Check sheet for the modelled part. Datum: model origin and axes. Units: mm. Face numbers are marked on the shaded views. A direction names the side the tool comes from. Give positions to 0.01 mm unless a question says otherwise; leave off trailing zeros. Loops run counter-clockwise (first coordinate to the right, second up) from the corner with the lowest first, then second, coordinate; pieces in that order, holes last. Notation, with made-up numbers: M -39.5,31.25 L -21.5,31.25 A20 cw -21.5,47.25 Z; hole C 31.25,-25.5 d1. An arc over 180 degrees is marked long. One line per question, with ' | ' between items. Start each with the question number.
from build123d import *

# Parameters (mm, degrees)
EXTRUDE_THIN1_DEPTH = 2.921
FILLET1_R           = 1.27
SKETCH2_W           = 6.858
SKETCH2_H           = 2.6035
CUT_EXTRUDE1_DEPTH  = 23.45746426


with BuildPart() as part:
    # Sketch1 → Extrude-Thin1 (new, symmetric)
    with BuildSketch(Plane(origin=(0, 0, 0), x_dir=(1, 0, 0), z_dir=(0, 1, 0))):
        with BuildLine():
            Line((0, 6.858), (0, 0))
            Line((0, 0), (0, -20.574))
            ThreePointArc((0, -20.574), (0.976529529, -21.809627404), (2.404370209, -21.145055365))
            Line((2.404370209, -21.145055365), (4.182370209, -17.613155736))
            ThreePointArc((4.182370209, -17.613155736), (4.283627404, -17.335570842), (4.318, -17.042100371))
            Line((4.318, -17.042100371), (4.318, -10.414))
            Line((4.318, -10.414), (3.81, -10.414))
            Line((3.81, -10.414), (3.81, -17.042100371))
            ThreePointArc((3.81, -17.042100371), (3.789376443, -17.218182654), (3.728622125, -17.38473359))
            Line((3.728622125, -17.38473359), (1.950622125, -20.916633219))
            ThreePointArc((1.950622125, -20.916633219), (1.093917717, -21.315376443), (0.508, -20.574))
            Line((0.508, -20.574), (0.508, 0))
            Line((0.508, 0), (0.508, 6.858))
            Line((0.508, 6.858), (0, 6.858))
        make_face()
    extrude(amount=EXTRUDE_THIN1_DEPTH, both=True)

    # Fillet1
    fillet1_edges = [part.edges().sort_by_distance(p)[0] for p in [
        (4.064, -2.921, 10.414),
        (4.064, 2.921, 10.414),
    ]]
    fillet(fillet1_edges, radius=FILLET1_R)

    # Sketch2 → Cut-Extrude1 (cut, through all)
    with BuildSketch(Plane.ZY):
        with Locations((-3.429, 1.61925)):
            Rectangle(SKETCH2_W, SKETCH2_H)
        with Locations((-3.429, -1.61925)):
            Rectangle(SKETCH2_W, SKETCH2_H)
    extrude(amount=-CUT_EXTRUDE1_DEPTH, mode=Mode.SUBTRACT)


solid = part.part
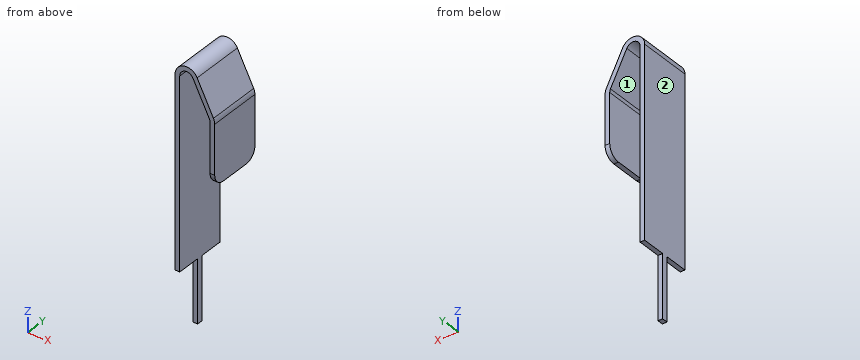
Q1. Depth check by flat-ended pin: P1, Ø2, axis at x = 3, y = -2, coming from the +Z side; P2, Ø0.6, axis at x = 0.5, z = -2, coming from the +Y side; P3, Ø0.6, axis at x = 0.5, y = -1.5, coming from the -Z side. Enter the tip coordinate at first touch or a pass-through.
Q2. Material ranges on probe 1 along X at (y, z) = (-0.15, 16.5); probe 2 along X at (y, z) = (-2.05, 5.75); probe 3 along Z at (x, y) = (1.2, 0.85), recorded low to high. Write a range as from..to.
Q3. Cross-section at C-C (z = 9.75). Record the cut outline in (x, y).
Q4. Cross-section at D-D (x = 1). Record the cut outline in (y, z), and give its area (3 significant figures).
Q5. Cross-section at B-B (y = 1.1). Record the cut outline in (x, z).
Q6. Access from +Z, -Z, +X, -X, +Y, -Y to the whole of each face (thin tool, end or side, straight path). Record for the marked faces 1 and 2.
Q7. Cross-section at A-A (z = 15.5). Record the cut outline in (x, y).
Solved:
1) P1: stops at z = 21.61 | P2: stops at y = 0.32 | P3: stops at z = 0
2) probe 1: x = 0..0.51, 3.81..4.32 | probe 2: x = 0..0.51 | probe 3: z = 21.33..21.84
3) outline: M 0,-2.92 L 0.51,-2.92 L 0.51,2.92 L 0,2.92 Z
4) outline: M -2.92,21.29 L 2.92,21.29 L 2.92,21.81 L -2.92,21.81 Z | area: 3.09 mm²
5) outline: M 0,0 L 0.51,0 L 0.51,20.57 A0.76 cw 1.95,20.92 L 3.73,17.38 A0.76 cw 3.81,17.04 L 3.81,10.41 L 4.32,10.41 L 4.32,17.04 A1.27 ccw 4.18,17.61 L 2.4,21.15 A1.27 ccw 0,20.57 Z
6) face 1: -Z, +Y, -Y | face 2: +Z, -Z, -X, +Y, -Y
7) outline: M 0,-2.92 L 0.51,-2.92 L 0.51,2.92 L 0,2.92 Z; M 3.81,-2.92 L 4.32,-2.92 L 4.32,2.92 L 3.81,2.92 Z
